from build123d import *

# Parameters (mm, degrees)
SKETCH2_W               = 88.9
SKETCH2_H               = 152.4
BOSS_EXTRUDE1_DEPTH     = 5.9944
SKETCH4_R               = 2.7305
CUT_EXTRUDE2_DEPTH      = 1
CUT_EXTRUDE2_DEPTH_BACK = 6.9944
SKETCH5_R               = 2.7305
CUT_EXTRUDE3_DEPTH      = 1
CUT_EXTRUDE3_DEPTH_BACK = 6.9944
SKETCH7_W               = 2.54
SKETCH7_H               = 152.4
CUT_EXTRUDE5_DEPTH      = 1
CUT_EXTRUDE5_DEPTH_BACK = 6.9944
SKETCH8_R               = 3.683
CUT_EXTRUDE6_DEPTH      = 4.064


with BuildPart() as part:
    # Sketch2 → Boss-Extrude1 (new body)
    with BuildSketch(Plane(origin=(0, 0, 0), x_dir=(1, 0, 0), z_dir=(0, 1, 0))):
        with Locations((44.45, 76.2)):
            Rectangle(SKETCH2_W, SKETCH2_H)
    extrude(amount=BOSS_EXTRUDE1_DEPTH)

    # Sketch4 → Cut-Extrude2 (cut, two sides)
    with BuildSketch(Plane(origin=(0, 5.9944, 0), x_dir=(1, 0, 0), z_dir=(0, 1, 0))) as cut_extrude2_sk:
        with Locations((45.72, 114.3)):
            Circle(SKETCH4_R)
        with Locations((45.72, 38.1)):
            Circle(SKETCH4_R)
    extrude(amount=CUT_EXTRUDE2_DEPTH, mode=Mode.SUBTRACT)
    extrude(cut_extrude2_sk.sketch, amount=-CUT_EXTRUDE2_DEPTH_BACK, mode=Mode.SUBTRACT)

    # Sketch5 → Cut-Extrude3 (cut, two sides)
    with BuildSketch(Plane(origin=(0, 5.9944, 0), x_dir=(1, 0, 0), z_dir=(0, 1, 0))) as cut_extrude3_sk:
        with Locations((69.85, 76.2)):
            Circle(SKETCH5_R)
        with Locations((19.05, 76.2)):
            Circle(SKETCH5_R)
        with Locations((44.45, 101.6)):
            Circle(SKETCH5_R)
        with Locations((44.45, 50.8)):
            Circle(SKETCH5_R)
    extrude(amount=CUT_EXTRUDE3_DEPTH, mode=Mode.SUBTRACT)
    extrude(cut_extrude3_sk.sketch, amount=-CUT_EXTRUDE3_DEPTH_BACK, mode=Mode.SUBTRACT)

    # Sketch7 → Cut-Extrude5 (cut, two sides)
    with BuildSketch(Plane(origin=(0, 5.9944, 0), x_dir=(1, 0, 0), z_dir=(0, 1, 0))) as cut_extrude5_sk:
        with Locations((1.27, 76.2)):
            Rectangle(SKETCH7_W, SKETCH7_H)
    extrude(amount=CUT_EXTRUDE5_DEPTH, mode=Mode.SUBTRACT)
    extrude(cut_extrude5_sk.sketch, amount=-CUT_EXTRUDE5_DEPTH_BACK, mode=Mode.SUBTRACT)

    # Sketch8 → Cut-Extrude6 (cut)
    with BuildSketch(Plane.XZ):
        with Locations((19.05, -76.2)):
            Circle(SKETCH8_R)
        with Locations((44.45, -50.8)):
            Circle(SKETCH8_R)
        with Locations((69.85, -76.2)):
            Circle(SKETCH8_R)
        with Locations((44.45, -101.6)):
            Circle(SKETCH8_R)
    extrude(amount=-CUT_EXTRUDE6_DEPTH, mode=Mode.SUBTRACT)


solid = part.part
Geometry: final body of the model. Coordinates: model frame, mm. A direction names the side the tool comes from. Round coordinates to 2 decimals unless told otherwise and drop trailing zeros. Loops run counter-clockwise (first coordinate to the right, second up) from the corner with the lowest first, then second, coordinate; pieces in that order, holes last.
Q1. Access query for faces 5 (the cylindrical face through (72.454, 5.043, -77.02)), 6 (the cylindrical face through (73.36, 2, -75.09)). Directions: +Z, -Z, +X, -X, +Y, -Y. A direction counts if a zero-diameter tool reaches every point of the face in a straight line with its end or side. Return the directions, or none.
Q2. Pull-direction query (Z, two-part tool) for faces 1 (the flat face through (45, 5.994, -77)), 2 (the cylindrical face through (45.71, 5.043, -99.178)), 3 (the cylindrical face through (20.52, 5.04, -78.5)), 4 (the flat face through (45, 3, 0)); classes: released by +Z, released by -Z, zero draft, split by the parting line, or undercut.
Q3. Section A-A on y = 2.8. Return loops of the section in (x, z).
Q4. Material intervals for L1, parallel to X at y = 0.65, z = -38; L2, parallel to Z at x = 44.45, y = 1.05, sorted ascending.
Q5. Pin query (flat end, axial travel): P1, Ø6, axis at x = 44.45, z = -101.6, coming from the -Y side. Return the tip coordinate at first contact, or that it passes through.
Q6. Section C-C on x = 69.85. Return loops of the section in (y, z).
Q7. Section B-B on z = -114.3. Return loops of the section in (x, y), plus the area to 3 significant figures.
Q8. Section D-D on z = -76.2. Return loops of the section in (x, y), plus the area to 3 significant figures.
Evaluation:
1. face 5: +Y, -Y
1. face 6: -Y
2. face 1: zero draft
2. face 2: undercut
2. face 3: undercut
2. face 4: released by +Z
3. outline: (2.54, -152.4) - (88.9, -152.4) - (88.9, 0) - (2.54, 0) - close; hole circle Ø7.37 at (19.05, -76.2); hole circle Ø7.37 at (44.45, -101.6); hole circle Ø7.37 at (44.45, -50.8); hole circle Ø5.46 at (45.72, -114.3); hole circle Ø5.46 at (45.72, -38.1); hole circle Ø7.37 at (69.85, -76.2)
4. L1: x = 2.54 to 42.99, 48.45 to 88.9
4. L2: z = -152.4 to -116.72, -111.88 to -105.28, -97.92 to -54.48, -47.12 to -40.52, -35.68 to 0
5. P1: stops at y = 4.06
6. outline: (0, -152.4) - (5.99, -152.4) - (5.99, -78.93) - (4.06, -78.93) - (4.06, -79.88) - (0, -79.88) - close; (0, -72.52) - (4.06, -72.52) - (4.06, -73.47) - (5.99, -73.47) - (5.99, 0) - (0, 0) - close
7. outline: (2.54, 0) - (42.99, 0) - (42.99, 5.99) - (2.54, 5.99) - close; (48.45, 0) - (88.9, 0) - (88.9, 5.99) - (48.45, 5.99) - close
7. area: 485 mm2
8. outline: (2.54, 0) - (15.37, 0) - (15.37, 4.06) - (16.32, 4.06) - (16.32, 5.99) - (2.54, 5.99) - close; (21.78, 4.06) - (22.73, 4.06) - (22.73, 0) - (66.17, 0) - (66.17, 4.06) - (67.12, 4.06) - (67.12, 5.99) - (21.78, 5.99) - close; (72.58, 4.06) - (73.53, 4.06) - (73.53, 0) - (88.9, 0) - (88.9, 5.99) - (72.58, 5.99) - close
8. area: 437 mm2
